Read the model definition and answer for the solid it produces. Units are mm, in the model's axes. Face numbers are marked on the shaded views. A direction names the side the tool comes from. Give positions to 0.01 mm unless a question says otherwise; leave off trailing zeros. Write each loop counter-clockwise with the first axis right and the second up, starting at its lowest first coordinate (ties: lowest second). Pieces come first, ordered by that corner, then holes.
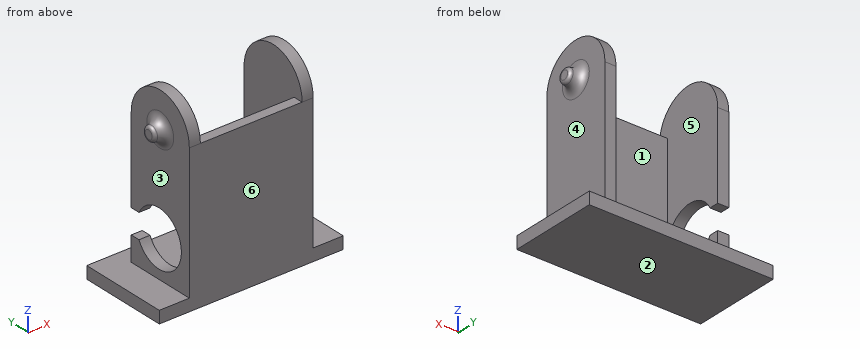
```python
from build123d import *

# Parameters (mm, degrees)
SKETCH1_W           = 20.2
SKETCH1_H           = 12
BOSS_EXTRUDE1_DEPTH = 1.6
BOSS_EXTRUDE2_DEPTH = 1.8
SKETCH3_R           = 1.2
BOSS_EXTRUDE3_DEPTH = 1.9
FILLET1_R           = 1.5
FILLET2_R           = 0.5
FILLET3_R           = 1.5
FILLET4_R           = 0.5
BOSS_EXTRUDE4_DEPTH = 10
SKETCH5_W           = 30
SKETCH5_H           = 17.5
BOSS_EXTRUDE5_DEPTH = 2
CUT_EXTRUDE1_DEPTH  = 2
SKETCH8_W           = 30
SKETCH8_H           = 2.9
CUT_EXTRUDE3_DEPTH  = 2


with BuildPart() as part:
    # Sketch1 → Boss-Extrude1 (new body)
    with BuildSketch(Plane(origin=(0, 0, 0), x_dir=(1, 0, 0), z_dir=(0, 1, 0))):
        Rectangle(SKETCH1_W, SKETCH1_H)
    extrude(amount=BOSS_EXTRUDE1_DEPTH)

    # Sketch2 → Boss-Extrude2 (add)
    with BuildSketch(Plane(origin=(10.1, 0, 0), x_dir=(0, 0, -1), z_dir=(1, 0, 0))):
        with BuildLine():
            Line((-6, 11.7), (6, 11.7))
            Line((6, 11.7), (6, 0))
            Line((6, 0), (-6, 0))
            ThreePointArc((-6, 0), (-11.85, 5.85), (-6, 11.7))
        make_face()
    boss_extrude2 = extrude(amount=-BOSS_EXTRUDE2_DEPTH)

    # Sketch3 → Boss-Extrude3 (add)
    with BuildSketch(Plane(origin=(10.1, 0, 0), x_dir=(0, 0, -1), z_dir=(1, 0, 0))):
        with Locations(Location((-6, 5.85, 0), (0, 0, 180))):
            Circle(SKETCH3_R)
    boss_extrude3 = extrude(amount=BOSS_EXTRUDE3_DEPTH)

    # Fillet1
    fillet1_edges = [part.edges().sort_by_distance(p)[0] for p in [
        (10.1, 5.85, 4.8),
    ]]
    fillet(fillet1_edges, radius=FILLET1_R)

    # Fillet2
    fillet2_edges = [part.edges().sort_by_distance(p)[0] for p in [
        (12, 5.85, 4.8),
    ]]
    fillet(fillet2_edges, radius=FILLET2_R)

    # Mirror2: Boss-Extrude2, Boss-Extrude3 across plane
    add(boss_extrude2.mirror(Plane(origin=(0, 0, 0), x_dir=(0, 0, 1), z_dir=(1, 0, 0))))
    add(boss_extrude3.mirror(Plane(origin=(0, 0, 0), x_dir=(0, 0, 1), z_dir=(1, 0, 0))))

    # Fillet3
    fillet3_edges = [part.edges().sort_by_distance(p)[0] for p in [
        (-10.1, 5.85, 4.8),
    ]]
    fillet(fillet3_edges, radius=FILLET3_R)

    # Fillet4
    fillet4_edges = [part.edges().sort_by_distance(p)[0] for p in [
        (-12, 5.85, 4.8),
    ]]
    fillet(fillet4_edges, radius=FILLET4_R)

    # Sketch4 → Boss-Extrude4 (add)
    with BuildSketch(Plane(origin=(0, 0, -6), x_dir=(-1, 0, 0), z_dir=(0, 0, -1))):
        Polygon((10.1, 0), (10.1, 11.7), (8.3, 11.7), (8.3, 1.6), (-8.3, 1.6), (-8.3, 11.7), (-10.1, 11.7), (-10.1, 0), align=None)
    extrude(amount=BOSS_EXTRUDE4_DEPTH)

    # Sketch5 → Boss-Extrude5 (add)
    with BuildSketch(Plane(origin=(0, 0, -16), x_dir=(-1, 0, 0), z_dir=(0, 0, -1))):
        with Locations((0, 5.85)):
            Rectangle(SKETCH5_W, SKETCH5_H)
    extrude(amount=BOSS_EXTRUDE5_DEPTH)

    # Sketch7 → Cut-Extrude1 (cut)
    with BuildSketch(Plane(origin=(-8.3, 0, 0), x_dir=(0, 0, -1), z_dir=(1, 0, 0))):
        with BuildLine():
            Line((8, 11.7), (12, 11.7))
            Line((12, 11.7), (12, 10.131128874))
            ThreePointArc((12, 10.131128874), (10, 1.6), (8, 10.131128874))
            Line((8, 10.131128874), (8, 11.7))
        make_face()
    extrude(amount=-CUT_EXTRUDE1_DEPTH, mode=Mode.SUBTRACT)

    # Sketch8 → Cut-Extrude3 (cut)
    with BuildSketch(Plane(origin=(0, 0, -18), x_dir=(-1, 0, 0), z_dir=(0, 0, -1))):
        with Locations((0, -1.45)):
            Rectangle(SKETCH8_W, SKETCH8_H)
    extrude(amount=-CUT_EXTRUDE3_DEPTH, mode=Mode.SUBTRACT)


solid = part.part
```
Item 1: Determine the mould class of the marked faces 3, 4, 5 and 6 for opening direction X: pulls with the +X half, pulls with the -X half, needs draft (parallel to the pull), parting line crosses it, or undercut.
Result set:
face 3: pulls with the -X half
face 4: pulls with the +X half
face 5: undercut
face 6: needs draft
Item 2: Find the intervals of material crossed by line 1 along Z through (x, y) = (-9.05, 6.1); line 2 along X through (y, z) = (8.5, -4.75); line 3 along Y through (x, z) = (-8.5, 1), in increasing order.
Result set:
line 1: z = -18 to -14.5, -5.5 to 11.84
line 2: x = -10.1 to -8.3, 8.3 to 10.1
line 3: y = 0 to 11.7
Item 3: Section D-D (z = -0.25) is taken. Write down the section's boundary in (x, y).
Result set:
outline: (-10.1, 0) - (10.1, 0) - (10.1, 11.7) - (8.3, 11.7) - (8.3, 1.6) - (-8.3, 1.6) - (-8.3, 11.7) - (-10.1, 11.7) - close
Item 4: Section C-C (x = 9.25) is taken. Write down the section's boundary in (y, z).
Result set:
outline: (0, -18) - (14.6, -18) - (14.6, -16) - (11.7, -16) - (11.7, 6) arc R5.85 ccw to (0, 6) - close
Item 5: Section A-A (z = -6) is taken. Write down the section's boundary in (x, y).
Result set:
outline: (-10.1, 0) - (10.1, 0) - (10.1, 11.7) - (8.3, 11.7) - (8.3, 1.6) - (-8.3, 1.6) - (-8.3, 4.04) - (-10.1, 4.04) - close; (-10.1, 8.16) - (-8.3, 8.16) - (-8.3, 11.7) - (-10.1, 11.7) - close
Item 6: Which of the six approach directions +Z, -Z, +X, -X, +Y, -Y give full straight-line access (tool end or side, diameter ignored) to the marked faces 1 and 2?
Result set:
face 1: +Z, +Y
face 2: -Z, +X, -X, +Y, -Y
Item 7: Section B-B (y = 9.5) is taken. Write down the section's boundary in (x, z).
Result set:
outline: (-15, -18) - (15, -18) - (15, -16) - (10.1, -16) - (10.1, 10.57) - (8.3, 10.57) - (8.3, -16) - (-8.3, -16) - (-8.3, -12.95) - (-10.1, -12.95) - (-10.1, -16) - (-15, -16) - close; (-10.1, -7.05) - (-8.3, -7.05) - (-8.3, 10.57) - (-10.1, 10.57) - close
Item 8: Each of these flat-tipped pins is pushed along its axis until it touches: pin 1 Ø3 at (x, y) = (-9.5, 8.5) entering from +Z; pin 2 Ø0.9 at (x, z) = (-9, -1) entering from +Y; pin 3 Ø0.7 at (y, z) = (5.5, 6) entering from +X. Where does it stop, or does it pass through?
Result set:
pin 1: stops at z = 11.74
pin 2: stops at y = 11.7
pin 3: stops at x = 12
